Verification items for the finished model (mm, model axes). Face numbers are marked on the shaded views. A direction names the side the tool comes from. Coordinates: 2 decimals unless noted, no trailing zeros. Write each loop counter-clockwise with the first axis right and the second up, starting at its lowest first coordinate (ties: lowest second). Pieces come first, ordered by that corner, then holes. Notation, with made-up numbers: (-29.5, 9) -> (-25.5, 9) arc R9 ccw to (-25.5, 16) -> close; hole circle Ø4 at (73.5, -33.5). An arc over 180 degrees is marked (long way). Use CSV: the item, a comma, the result in double quotes.
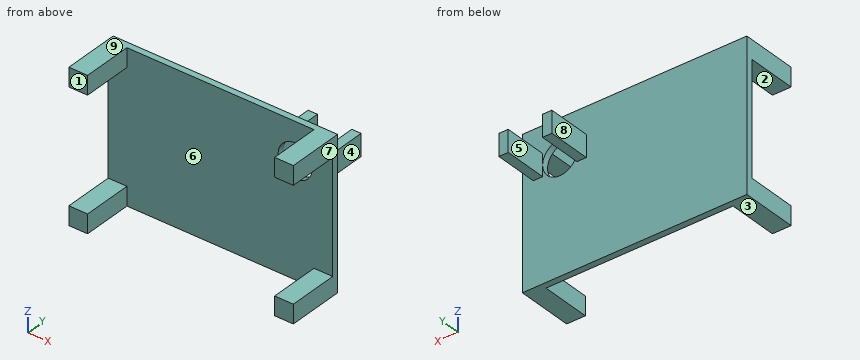
```python
from build123d import *

# Parameters (mm, degrees)
SKETCH1_W           = 914.4
SKETCH1_H           = 609.6
BOSS_EXTRUDE2_DEPTH = 25.4
SKETCH1_3_R         = 69.85
CUT_EXTRUDE2_DEPTH  = 1100.265518426
SKETCH1_4_W         = 38.1
SKETCH1_4_H         = 88.9
BOSS_EXTRUDE3_DEPTH = 203.2
SKETCH3_W           = 76.2
SKETCH3_H           = 76.2
BOSS_EXTRUDE4_DEPTH = 203.2


with BuildPart() as part:
    # Sketch1 → Boss-Extrude2 (new body)
    with BuildSketch(Plane(origin=(0, 0, 0), x_dir=(1, 0, 0), z_dir=(0, 1, 0))):
        with Locations((457.2, 304.8)):
            Rectangle(SKETCH1_W, SKETCH1_H)
    extrude(amount=BOSS_EXTRUDE2_DEPTH)

    # Sketch1_3 → Cut-Extrude2 (cut, through all)
    with BuildSketch(Plane(origin=(0, 0, 0), x_dir=(1, 0, 0), z_dir=(0, 1, 0))):
        with Locations(Location((762, 152.4, 0), (0, 0, 270))):
            Circle(SKETCH1_3_R)
    extrude(amount=CUT_EXTRUDE2_DEPTH, mode=Mode.SUBTRACT)

    # Sketch1_4 → Boss-Extrude3 (add)
    with BuildSketch(Plane(origin=(0, 0, 0), x_dir=(1, 0, 0), z_dir=(0, 1, 0))):
        with Locations((673.1, 152.4)):
            Rectangle(SKETCH1_4_W, SKETCH1_4_H)
        with Locations((850.9, 152.4)):
            Rectangle(SKETCH1_4_W, SKETCH1_4_H)
    extrude(amount=BOSS_EXTRUDE3_DEPTH)

    # Sketch3 → Boss-Extrude4 (add)
    with BuildSketch(Plane.XZ):
        with Locations((38.1, -571.5)):
            Rectangle(SKETCH3_W, SKETCH3_H)
        with Locations((38.1, -38.1)):
            Rectangle(SKETCH3_W, SKETCH3_H)
        with Locations((876.3, -571.5)):
            Rectangle(SKETCH3_W, SKETCH3_H)
        with Locations((876.3, -38.1)):
            Rectangle(SKETCH3_W, SKETCH3_H)
    extrude(amount=BOSS_EXTRUDE4_DEPTH)


solid = part.part
```
1) Gauge pin test, flat ends, axial feed: pin 1 (4 mm diameter, centred on x = 457, z = -340, fed in from +Y); pin 2 (10 mm diameter, centred on x = 466.5, z = -120.5, fed in from -Y). Record the tip position at first contact, or that the pin passes through.
Return value:
pin 1,"y = 25.4"
pin 2,"y = 0"
2) Cross-section at D-D (z = -142). Record the boundary of the cut face in (x, y).
Return value:
outline,"(0, 0) -> (692.93, 0) -> (692.93, 25.4) -> (692.15, 25.4) -> (692.15, 203.2) -> (654.05, 203.2) -> (654.05, 25.4) -> (0, 25.4) -> close; (831.07, 0) -> (914.4, 0) -> (914.4, 25.4) -> (869.95, 25.4) -> (869.95, 203.2) -> (831.85, 203.2) -> (831.85, 25.4) -> (831.07, 25.4) -> close"
3) Mould release check, pull along X, two halves, no side actions. Record for the marked faces 6, 7, 8 and 9: released by +X, released by -X, zero draft, split by the parting line, or undercut.
Return value:
face 6,"undercut"
face 7,"released by +X"
face 8,"released by -X"
face 9,"zero draft"
4) Scan lines: L1, parallel to X at y = 179.5, z = -188; L2, parallel to Z at x = 762, y = 11.25; L3, parallel to Y at x = 644, z = -167. Record each from-to range of solid material in increasing order.
Return value:
L1,"654.05 to 692.15, 831.85 to 869.95"
L2,"-609.6 to -222.25, -82.55 to 0"
L3,"0 to 25.4"
5) Cross-section at A-A (y = -63.5). Record the boundary of the cut face in (x, z), plus the area to 3 significant figures.
Return value:
outline,"(0, -609.6) -> (76.2, -609.6) -> (76.2, -533.4) -> (0, -533.4) -> close; (0, -76.2) -> (76.2, -76.2) -> (76.2, 0) -> (0, 0) -> close; (838.2, -609.6) -> (914.4, -609.6) -> (914.4, -533.4) -> (838.2, -533.4) -> close; (838.2, -76.2) -> (914.4, -76.2) -> (914.4, 0) -> (838.2, 0) -> close"
area,"23,200 mm2"
6) Set-up check for the marked faces 1, 2, 3, 4 and 5: record each of +Z, -Z, +X, -X, +Y, -Y from which the full face is reachable in a straight line by a thin tool's end or side.
Return value:
face 1,"+Z, -Z, +X, -X, -Y"
face 2,"+X, -X, -Y"
face 3,"-Z, +X, -X, +Y, -Y"
face 4,"+Z, -Z, +X, +Y"
face 5,"+Z, -Z, +Y"
7) Cross-section at B-B (x = 762). Record the boundary of the cut face in (y, z).
Return value:
outline,"(0, -609.6) -> (25.4, -609.6) -> (25.4, -222.25) -> (0, -222.25) -> close; (0, -82.55) -> (25.4, -82.55) -> (25.4, 0) -> (0, 0) -> close"
8) Cross-section at C-C (y = 144). Record the boundary of the cut face in (x, z).
Return value:
outline,"(654.05, -196.85) -> (692.15, -196.85) -> (692.15, -107.95) -> (654.05, -107.95) -> close; (831.85, -196.85) -> (869.95, -196.85) -> (869.95, -107.95) -> (831.85, -107.95) -> close"
